Part print with two shaded views. Sizes in mm from the minimum x, y, z corner. Coordinates: 2 decimals unless noted, no trailing zeros. Order: outer loops, then holes, each group sorted by start corner. A loop starts at its lowest first (then second) coordinate and runs counter-clockwise, first axis right, second up.
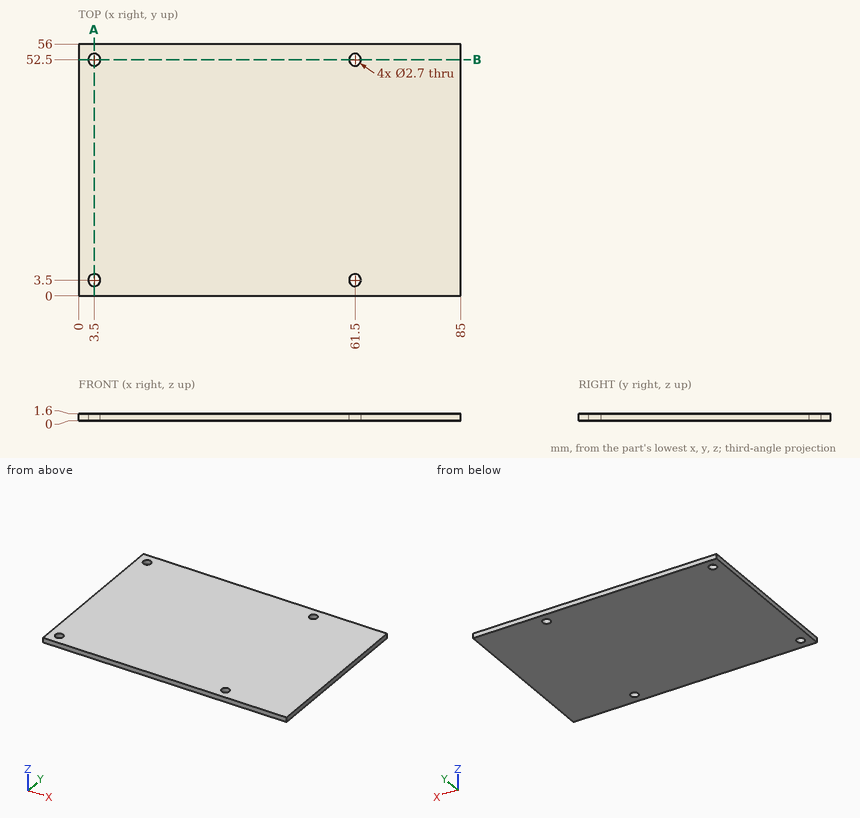
Q1. Pin check, flat tips, straight feed: pin 1 Ø2.5 at (x, y) = (3.5, 3.5) entering from +Z; pin 2 Ø3 at (x, y) = (55.5, 15) entering from -Z. Stop position of each tip, or through.
Results list:
pin 1: passes through
pin 2: stops at z = 0
Q2. Wall check: line 1 along Y through (x, z) = (3.5, 0.4); line 2 along X through (y, z) = (52, 1.45). Give the ranges that are in metal, low to high.
Results list:
line 1: y = 0 to 2.15, 4.85 to 51.15, 53.85 to 56
line 2: x = 0 to 2.25, 4.75 to 60.25, 62.75 to 85
Q3. Cut at B-B on y = 52.5. Write the cut outline in (x, z).
Results list:
outline: (0, 0) - (2.15, 0) - (2.15, 1.6) - (0, 1.6) - close; (4.85, 0) - (60.15, 0) - (60.15, 1.6) - (4.85, 1.6) - close; (62.85, 0) - (85, 0) - (85, 1.6) - (62.85, 1.6) - close
Q4. Cut at A-A on x = 3.5. Write the cut outline in (y, z), and give its area (3 significant figures).
Results list:
outline: (0, 0) - (2.15, 0) - (2.15, 1.6) - (0, 1.6) - close; (4.85, 0) - (51.15, 0) - (51.15, 1.6) - (4.85, 1.6) - close; (53.85, 0) - (56, 0) - (56, 1.6) - (53.85, 1.6) - close
area: 81.0 mm2
